from build123d import *

# Parameters (mm, degrees)
F1_DEPTH     = 1
F2_DEPTH     = 11
F4_DEPTH     = 88.001
F5_T         = 1
F5_T3_DEPTH  = 130
F5_T5_DEPTH  = 60
F5_T8_ANGLE  = 90.000000001
F5_T10_ANGLE = 90.000000001
F5_T12_ANGLE = 90.000000001
F5_T14_ANGLE = 90.000000001
F8_DEPTH     = 10


# Not quite as in the source:
# - a shell that OpenCascade refuses in one call is made with other operations: the cavity is built on its own and cut out


with BuildPart() as f1:
    # F0 (on Top) → F1 (new body)
    with BuildSketch(Plane.XY):
        with BuildLine():
            ThreePointArc((0, 15), (4.3933982822, 4.3933982822), (15, 0))
            Line((15, 0), (143, 0))
            ThreePointArc((143, 0), (153.6066017178, 4.3933982822), (158, 15))
            Line((158, 15), (158, 73))
            ThreePointArc((158, 73), (153.6066017178, 83.6066017178), (143, 88))
            Line((143, 88), (15, 88))
            ThreePointArc((15, 88), (4.3933982822, 83.6066017178), (0, 73))
            Line((0, 73), (0, 15))
        make_face()
        with BuildLine():
            ThreePointArc((1.5, 73), (5.454058454, 82.545941546), (15, 86.5))
            Line((15, 86.5), (143, 86.5))
            ThreePointArc((143, 86.5), (152.545941546, 82.545941546), (156.5, 73))
            Line((156.5, 73), (156.5, 15))
            ThreePointArc((156.5, 15), (152.545941546, 5.454058454), (143, 1.5))
            Line((143, 1.5), (15, 1.5))
            ThreePointArc((15, 1.5), (5.454058454, 5.454058454), (1.5, 15))
            Line((1.5, 15), (1.5, 73))
        make_face(mode=Mode.SUBTRACT)
    extrude(amount=F1_DEPTH)

    # F0 (on Top) → F2 (join)
    with BuildSketch(Plane.XY):
        with BuildLine():
            Line((143, 86.5), (15, 86.5))
            ThreePointArc((15, 86.5), (5.454058454, 82.545941546), (1.5, 73))
            Line((1.5, 73), (1.5, 15))
            ThreePointArc((1.5, 15), (5.454058454, 5.454058454), (15, 1.5))
            Line((15, 1.5), (143, 1.5))
            ThreePointArc((143, 1.5), (152.545941546, 5.454058454), (156.5, 15))
            Line((156.5, 15), (156.5, 73))
            ThreePointArc((156.5, 73), (152.545941546, 82.545941546), (143, 86.5))
        make_face()
    extrude(amount=F2_DEPTH)

    # F3 (on Front) → F4 (cut, through all)
    with BuildSketch(Plane.XZ):
        with BuildLine():
            ThreePointArc((0, 6.0560618341), (7.3283980564, 9.4088283813), (15.2286913721, 11))
            ThreePointArc((15.2286913721, 11), (15.6141911349, 11.030157259), (16, 11.0560618341))
            Line((16, 11.0560618341), (0, 11.0560618341))
            Line((0, 11.0560618341), (0, 6.0560618341))
        make_face()
        with BuildLine():
            ThreePointArc((142, 11.0560618341), (142.3858088651, 11.030157259), (142.7713086279, 11))
            ThreePointArc((142.7713086279, 11), (150.6716019436, 9.4088283813), (158, 6.0560618341))
            Line((158, 6.0560618341), (158, 11.0560618341))
            Line((158, 11.0560618341), (142, 11.0560618341))
        make_face()
    extrude(amount=-F4_DEPTH, mode=Mode.SUBTRACT)

    # F5: shell of thickness 1, made by hand


with BuildPart() as f5_core1:
    # F5_t2: copy of F1
    add(f1.part)

    # the walls: a layer under each face that stays
    f5_faces = [f5_core1.faces().sort_by_distance(p)[0] for p in [
        (0, 44, 0.5),
        (4.3933982822, 83.6066017178, 0.5),
        (4.3933982822, 4.3933982822, 0.5),
        (133.3125, 1.0864197531, 1),
        (79, 88, 0.5),
        (79, 0, 0.5),
        (153.6066017178, 4.3933982822, 0.5),
        (158, 44, 0.5),
        (153.6066017178, 83.6066017178, 0.5),
        (5.454058454, 82.545941546, 5.9900432581),
        (79, 86.5, 6),
        (152.545941546, 82.545941546, 5.9900432581),
        (156.5, 44, 3.9570518678),
        (152.545941546, 5.454058454, 5.9900432581),
        (79, 1.5, 6),
        (5.454058454, 5.454058454, 5.9900432581),
        (1.5, 44, 3.9570518678),
        (8.1534990202, 44, 9.6655007895),
        (79, 44, 11),
        (149.8465009798, 44, 9.6655007895),
    ]]
    thicken(f5_faces, amount=-F5_T, mode=Mode.SUBTRACT)

    # F5_s4 → F5_t3 (cut)
    with BuildSketch(Plane.YZ.offset(14)):
        Polygon((86.51, 1.01), (86.5, 0), (85.5, 0), (85.5, 1), align=None)
        Polygon((1.49, 1.01), (1.5, 0), (2.5, 0), (2.5, 1), align=None)
    extrude(amount=F5_T3_DEPTH, mode=Mode.SUBTRACT)

    # F5_s6 → F5_t5 (cut)
    with BuildSketch(Plane.XZ.offset(-74)):
        Polygon((156.51, 1.01), (156.5, 0), (155.5, 0), (155.5, 1), align=None)
        Polygon((1.49, 1.01), (1.5, 0), (2.5, 0), (2.5, 1), align=None)
    extrude(amount=F5_T5_DEPTH, mode=Mode.SUBTRACT)

    # F5_s7 → F5_t8 (revolve, cut)
    with BuildSketch(Plane.XZ.offset(-73)):
        Polygon((1.49, 1.01), (1.5, 0), (2.5, 0), (2.5, 1), align=None)
    revolve(axis=Axis((15, 73, 1), (0, 0, -1)), revolution_arc=F5_T8_ANGLE, mode=Mode.SUBTRACT)

    # F5_s9 → F5_t10 (revolve, cut)
    with BuildSketch(Plane.YZ.offset(143)):
        Polygon((86.51, 1.01), (86.5, 0), (85.5, 0), (85.5, 1), align=None)
    revolve(axis=Axis((143, 73, 1), (0, 0, -1)), revolution_arc=F5_T10_ANGLE, mode=Mode.SUBTRACT)

    # F5_s11 → F5_t12 (revolve, cut)
    with BuildSketch(Plane.XZ.offset(-15)):
        Polygon((156.51, 1.01), (156.5, 0), (155.5, 0), (155.5, 1), align=None)
    revolve(axis=Axis((143, 15, 1), (0, 0, -1)), revolution_arc=F5_T12_ANGLE, mode=Mode.SUBTRACT)

    # F5_s13 → F5_t14 (revolve, cut)
    with BuildSketch(Plane.YZ.offset(15)):
        Polygon((1.49, 1.01), (1.5, 0), (2.5, 0), (2.5, 1), align=None)
    revolve(axis=Axis((15, 15, 1), (0, 0, -1)), revolution_arc=F5_T14_ANGLE, mode=Mode.SUBTRACT)


with BuildPart() as f1_1:
    add(f1.part)

    # what is left inside the walls is the cavity
    f5_cavity = [f5_core1.part.solids().sort_by_distance(p)[0] for p in [
        (79, 30.166667, 0.01),
    ]]
    add(f5_cavity, mode=Mode.SUBTRACT)

    # F6 (on Top) → F7 (join, up to the next surface of F1)
    with BuildSketch(Plane.XY):
        with BuildLine():
            Line((143, 83.5), (15, 83.5))
            ThreePointArc((15, 83.5), (7.5753787975, 80.4246212025), (4.5, 73))
            Line((4.5000000324, 73), (4.5000000324, 14.9847623929))
            ThreePointArc((4.5000000324, 14.9847623929), (7.5753788898, 7.5753631149), (14.9847847018, 4.5))
            Line((14.9847847018, 4.5), (143, 4.5))
            ThreePointArc((143, 4.5), (150.4246212025, 7.5753787975), (153.5, 15))
            Line((153.5, 15), (153.5, 73))
            ThreePointArc((153.5, 73), (150.4246212025, 80.4246212025), (143, 83.5))
        make_face()
    extrude(until=Until.NEXT)

    # F6 (on Top) → F8 (join)
    with BuildSketch(Plane.XY):
        with BuildLine():
            Line((143, 83.5), (15, 83.5))
            ThreePointArc((15, 83.5), (7.5753787975, 80.4246212025), (4.5, 73))
            Line((4.5000000324, 73), (4.5000000324, 14.9847623929))
            ThreePointArc((4.5000000324, 14.9847623929), (7.5753788898, 7.5753631149), (14.9847847018, 4.5))
            Line((14.9847847018, 4.5), (143, 4.5))
            ThreePointArc((143, 4.5), (150.4246212025, 7.5753787975), (153.5, 15))
            Line((153.5, 15), (153.5, 73))
            ThreePointArc((153.5, 73), (150.4246212025, 80.4246212025), (143, 83.5))
        make_face()
    extrude(amount=-F8_DEPTH)


solid = f1_1.part
For this review, take the finished solid that the model builds, in its own axes (mm). A direction names the side the tool comes from. Round coordinates to 2 decimals unless told otherwise and drop trailing zeros. Write each loop counter-clockwise with the first axis right and the second up, starting at its lowest first coordinate (ties: lowest second). Pieces come first, ordered by that corner, then holes. Notation, with made-up numbers: (-36, -38.5) -> (23, -38.5) arc R12 ccw to (23, -16.5) -> close; hole circle Ø10 at (-36.75, -23.5). An arc over 180 degrees is marked (long way). Put each result on its own line as item: value.
Q1. Consider section C-C on y = 66.5. State the section outline as (x, z) points.
Determined:
outline: (0, 0) -> (2.5, 0) -> (2.5, 6.31) arc R34.07 cw to (4.5, 7.27) -> (4.5, -10) -> (153.5, -10) -> (153.5, 7.27) arc R34.07 cw to (155.5, 6.31) -> (155.5, 0) -> (158, 0) -> (158, 1) -> (156.5, 1) -> (156.5, 6.91) arc R35.07 ccw to (142.77, 11) -> (15.23, 11) arc R35.07 ccw to (1.5, 6.91) -> (1.5, 1) -> (0, 1) -> close
Q2. To check wall thickness, follow L1, parallel to Y at x = 41.5, z = 5.75; L2, parallel to Y at x = 128.5, z = 0.5; L3, parallel to X at y = 43, z = 3. State the ranges of each line that lie inside material, in increasing order. Write a range as [from, to].
Determined:
L1: y = [1.5, 2.5], [4.5, 83.5], [85.5, 86.5]
L2: y = [0, 2.5], [4.5, 83.5], [85.5, 88]
L3: x = [1.5, 2.5], [4.5, 153.5], [155.5, 156.5]
Q3. Consider section B-B on x = 64.5. State the section outline as (y, z) points, and give its area (3 significant figures).
Determined:
outline: (0, 0) -> (2.5, 0) -> (2.5, 10) -> (4.5, 10) -> (4.5, -10) -> (83.5, -10) -> (83.5, 10) -> (85.5, 10) -> (85.5, 0) -> (88, 0) -> (88, 1) -> (86.5, 1) -> (86.5, 11) -> (1.5, 11) -> (1.5, 1) -> (0, 1) -> close
area: 1,690 mm^2
Q4. Consider section A-A on z = -6.5. State the section outline as (x, y) points, and give its area (3 significant figures).
Determined:
outline: (4.5, 14.98) arc R10.5 ccw to (14.98, 4.5) -> (143, 4.5) arc R10.5 ccw to (153.5, 15) -> (153.5, 73) arc R10.5 ccw to (143, 83.5) -> (15, 83.5) arc R10.5 ccw to (4.5, 73) -> close
area: 11,700 mm^2
Q5. Machinability: for faces 1 (the flat face through (153.5, 44, -1)), 2 (the flat face through (80, 86.5, 6)), 3 (the flat face through (1.5, 44, 4)), 4 (the cylindrical face through (7.136, 4.027, 4.811)), 5 (the cylindrical face through (150.864, 83.973, 4.811)), which of the approach directions +Z, -Z, +X, -X, +Y, -Y give a long, thin tool a straight path to every point of the face, cutting with its end or side? Answer none if there is none.
Determined:
face 1: -Z
face 2: +Z, +X, -X, +Y
face 3: +Z, -X, +Y, -Y
face 4: +Z, -X, -Y
face 5: +Z, +X, +Y
Q6. Consider section D-D on y = 77. State the section outline as (x, z) points, and give its area (3 significant figures).
Determined:
outline: (0.54, 0) -> (3.16, 0) -> (3.16, 6.64) arc R34.07 cw to (5.29, 7.6) -> (5.29, -10) -> (152.71, -10) -> (152.71, 7.6) arc R34.07 cw to (154.84, 6.64) -> (154.84, 0) -> (157.46, 0) -> (157.46, 1) -> (155.89, 1) -> (155.89, 7.23) arc R35.07 ccw to (142.77, 11) -> (15.23, 11) arc R35.07 ccw to (2.11, 7.23) -> (2.11, 1) -> (0.54, 1) -> close
area: 3,100 mm^2
Q7. Clearance check with flat-ended pins moving along their axes: pin 1 Ø8 at (x, z) = (91, 8.5) entering from +Y; pin 2 Ø2 at (y, z) = (74, -3) entering from +X; pin 3 Ø10 at (y, z) = (25, 6.5) entering from +X. State where each tip first meets the part, or that it passes through.
Determined:
pin 1: stops at y = 86.5
pin 2: stops at x = 153.5
pin 3: stops at x = 156.5
